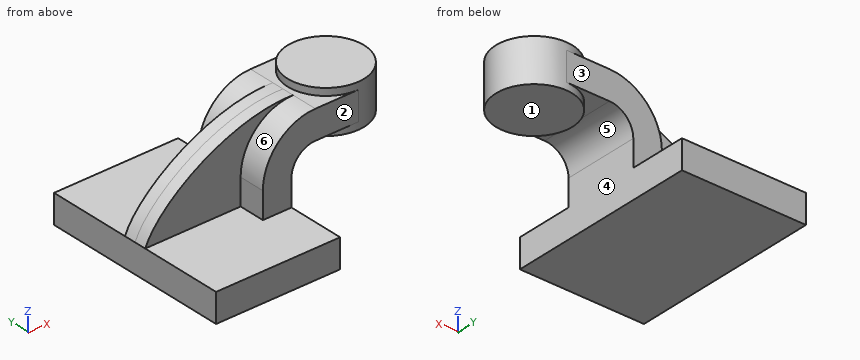
from build123d import *

# Parameters (mm, degrees)
F1_DEPTH = 63.5
F0_W     = 25.4
F0_H     = 19.05
F2_DEPTH = 25.4
F3_DEPTH = 7.9375


with BuildPart() as f1:
    # F0 (on Front) → F1 (new body, symmetric)
    with BuildSketch(Plane.XZ):
        Polygon((41.275, -9.525), (41.275, 9.525), (22.225, 9.525), (-41.275, 9.525), (-41.275, -9.525), align=None)
    extrude(amount=F1_DEPTH, both=True)

    # F0 (on Front) → F2 (join, symmetric)
    with BuildSketch(Plane.XZ):
        with BuildLine():
            Line((22.225, 9.525), (41.275, 9.525))
            Line((41.275, 9.525), (41.275, 27.0002))
            ThreePointArc((41.275, 27.0002), (45.9246798487, 38.2255201513), (57.15, 42.8752))
            Line((57.15, 42.8752), (60.325, 42.8752))
            Line((60.325, 42.8752), (60.325, 61.9252))
            Line((60.325, 61.9252), (57.15, 61.9252))
            ThreePointArc((57.15, 61.9252), (32.4542956671, 51.6959043329), (22.225, 27.0002))
            Line((22.225, 27.0002), (22.225, 9.525))
        make_face()
        with Locations((73.025, 52.4002)):
            Rectangle(F0_W, F0_H)
    extrude(amount=F2_DEPTH, both=True)

    # F0 (on Front) → F3 (join, symmetric)
    with BuildSketch(Plane.XZ):
        with BuildLine():
            Line((-41.275, 9.525), (22.225, 9.525))
            Line((22.225, 9.525), (22.225, 27.0002))
            ThreePointArc((22.225, 27.0002), (32.4542956671, 51.6959043329), (57.15, 61.9252))
            add(Edge.make_bspline(
                [(-41.275, 9.525), (-31.6697917879, 33.0327823758), (15.2440918609, 64.0094131231), (57.15, 61.9252)],
                knots=[0, 0, 0, 0, 111.5045361635, 111.5045361635, 111.5045361635, 111.5045361635], degree=3))
        make_face()
    extrude(amount=F3_DEPTH, both=True)

    # F0 (on Front) → F4 (revolve)
    with BuildSketch(Plane.XZ):
        Polygon((85.725, 61.9252), (85.725, 42.8752), (85.725, 38.1), (111.125, 38.1), (111.125, 66.675), (85.725, 66.675), align=None)
    revolve(axis=Axis((85.725, 0, 52.3875), (0, 0, -1)))


solid = f1.part
The listing builds one solid part. Answer for the finished solid, in the listing's coordinates (mm). Face numbers are marked on the shaded views. A direction names the side the tool comes from. Give positions to 0.01 mm unless a question says otherwise; leave off trailing zeros. Write each loop counter-clockwise with the first axis right and the second up, starting at its lowest first coordinate (ties: lowest second). Pieces come first, ordered by that corner, then holes.
Item 1: Which of the six approach directions +Z, -Z, +X, -X, +Y, -Y give full straight-line access (tool end or side, diameter ignored) to the marked faces 1, 2 and 3?
Item 2: Section A-A, the plane y = -49 is taken. Write down the section's boundary in (x, z) (3 decimals).
Item 3: Determine the mould class of the marked faces 4, 5 and 6 for opening direction X: released by +X, released by -X, zero draft, split by the parting line, or undercut.
Item 4: Find the intervals of material crossed by line 1 along X through (y, z) = (5.5, 1) (3 decimals); line 2 along X through (y, z) = (-15, 20) (3 decimals); line 3 along Z through (x, y) = (71.5, -6) (3 decimals), in increasing order.
Item 5: Section B-B, the plane z = -3 is taken. Write down the section's boundary in (x, y) (3 decimals).
Item 6: Flat-ended cylindrical pins translate along their axes: P1, Ø1, axis at x = 32.5, z = 16.5, coming from the -Y side; P2, Ø11, axis at y = -5, z = 7.5, coming from the +X side (3 decimals); P3, Ø19, axis at y = -14.5, z = 15.5, coming from the -X side (3 decimals); P4, Ø10, axis at y = 42.5, z = 19, coming from the +X side. Find the tip coordinate at first contact, or state that the pin passes through.
Item 7: Section C-C, the plane x = 62.5 is taken. Write down the section's boundary in (y, z) (3 decimals).
Item 8: Section D-D, the plane y = -20.5 is taken. Write down the section's boundary in (x, z) (3 decimals).
Completed:
1. face 1: -Z, +X, +Y, -Y
1. face 2: +Z, +X, -X, -Y
1. face 3: +Z, +X, -X, +Y
2. outline: (-41.275, -9.525) - (41.275, -9.525) - (41.275, 9.525) - (-41.275, 9.525) - close
3. face 4: released by +X
3. face 5: undercut
3. face 6: released by -X
4. line 1: x = -41.275 to 41.275
4. line 2: x = 22.225 to 41.275
4. line 3: z = 38.1 to 66.675
5. outline: (-41.275, -63.5) - (41.275, -63.5) - (41.275, 63.5) - (-41.275, 63.5) - close
6. P1: stops at y = -25.4
6. P2: stops at x = 41.275
6. P3: stops at x = -41.275
6. P4: passes through
7. outline: (-25.4, 42.875) - (-10.284, 42.875) - (-10.284, 38.1) - (10.284, 38.1) - (10.284, 42.875) - (25.4, 42.875) - (25.4, 61.925) - (10.284, 61.925) - (10.284, 66.675) - (-10.284, 66.675) - (-10.284, 61.925) - (-25.4, 61.925) - close
8. outline: (-41.275, -9.525) - (41.275, -9.525) - (41.275, 27) arc R15.875 cw to (57.15, 42.875) - (70.728, 42.875) - (70.728, 38.1) - (100.722, 38.1) - (100.722, 66.675) - (70.728, 66.675) - (70.728, 61.925) - (57.15, 61.925) arc R34.925 ccw to (22.225, 27) - (22.225, 9.525) - (-41.275, 9.525) - close
